Can you work these out from the model? Positions are in its coordinate system, mm. Face numbers are marked on the shaded views. A direction names the side the tool comes from. Coordinates: 2 decimals unless noted, no trailing zeros. Order: outer loops, then holes, each group sorted by start corner. A loop starts at its lowest first (then second) coordinate and runs counter-clockwise, first axis right, second up.
Autodesk Inventor part; units mm, degrees
ref_plane "Work Plane1" through (76.2, 0, 0) normal (1, 0, 0) x (0, 1, 0)
ref_plane "Work Plane4" through (63.5, 0, 0) normal (1, 0, 0) x (0, 1, 0)
ref_plane "XZ Plane" through (0, 0, 0) normal (0, 1, 0) x (-1, 0, 0)
sketch "Sketch1" plane through (0, 0, 0) normal (0, 0, 1) x (1, 0, 0)
  line L0 (107.721093, 0) -> (-76.2, 0)
  line L1 (-76.2, 0) -> (-76.2, -12.7)
  line L2 (-76.2, -12.7) -> (69.621093, -12.700026)
  line L3 (107.721093, -6.350016) -> (107.721093, 0)
  line L4 (107.721093, -6.350016) -> (69.621093, -12.700026)
  point P0 (0, 0)
  dimension "d19" = 183.92109
  dimension "d20" = 76.2
  dimension "d21" = 12.7
  dimension "d22" = 38.1
extrude "Extrusion2" add sketch "Sketch1" along normal blind 25.4
sketch "Sketch2" plane through (-76.2, 0, 0) normal (0, 1, 0) x (1, 0, 0)
  circle A0 centre (76.2, 0) radius 22.5
  dimension "d25" = 45
extrude "Extrusion3" cut sketch "Sketch2" against normal through all
mirror "Mirror1" about plane through (14.352169, -5.990033, 0) normal (0, 0, -1) of "Extrusion2", "Extrusion3"
sketch "Sketch4" plane through (-76.2, 0, 25.4) normal (0, 1, 0) x (1, 0, 0)
  circle A0 centre (38.1, 25.4) radius 3.81
  line L0 (-36.784219, 25.4) -> (220.705311, 25.4)
  point P0 (76.2, 25.4)
  dimension "d13" = 7.62
  dimension "d39" = 38.1
extrude "Extrusion5" add sketch "Sketch4" along normal blind 7.62
ref_plane "Work Plane1" through (76.2, 0, 0) normal (1, 0, 0) x (0, 1, 0)
sketch "Sketch10" plane through (69.621093, -12.700026, -25.4) normal (-0.0000002, -1, 0) x (1, -0.0000002, 0)
  line L0 (-69.621095, 36.62532) -> (38.099999, 36.62532)
  line L1 (-69.621095, 14.17468) -> (38.1, 14.17468)
  circle A0 centre (-69.621095, 25.4) radius 11.22532
  line L2 (-69.621095, 36.62532) -> (-69.621095, 14.17468) construction
  line L3 (38.099999, 0) -> (38.099999, 50.8) construction
  line L4 (38.099999, 36.62532) -> (38.1, 14.17468)
  point P0 (-69.621095, 25.4)
extrude "Extrusion11" cut sketch "Sketch10" against normal mid plane 15.24
ref_plane "Work Plane4" through (63.5, 0, 0) normal (1, 0, 0) x (0, 1, 0)
sketch "Sketch5" plane through (76.2, 0, 0) normal (1, 0, 0) x (0, 1, 0)
  line L0 (-1.5875, -10.237854) -> (9.525, -10.237854)
  line L1 (9.525, -10.237854) -> (9.525, 10.237854)
  line L2 (9.525, 10.237854) -> (-1.5875, 10.237854)
  line L3 (-1.5875, 10.237854) -> (-1.5875, -10.237854)
  line L4 (9.525, -7.62) -> (0, -7.62)
  line L5 (0, -7.62) -> (0, 7.62)
  line L6 (0, 7.62) -> (9.525, 7.62)
  line L7 (9.525, 7.62) -> (9.525, -7.62)
  line L8 (0, 25.4) -> (0, -25.4)
  line L9 (9.525, -7.62) -> (6.5, -7.62)
  line L10 (6.5, -7.62) -> (6.5, -4.62)
  line L11 (6.5, -4.62) -> (9.525, -4.62)
  line L12 (9.525, -4.62) -> (9.525, -7.62)
  line L13 (9.525, 7.62) -> (6.5, 7.62)
  line L14 (6.5, 7.62) -> (6.5, 4.62)
  line L15 (6.5, 4.62) -> (9.525, 4.62)
  line L16 (9.525, 4.62) -> (9.525, 7.62)
  point P0 (0, 0)
  point P1 (0, 0)
  point P2 (9.525, 0)
  dimension "d14" = 15.24
  dimension "d50" = 6.5
  dimension "d51" = 3
  dimension "d52" = 3
extrude "Extrusion6" add sketch "Sketch5" along normal blind 20 contours L3 L2 L8 L5 L0 | L8 L4 L1 L0 | L2 L1 L6 L8 | L4 L10 L11 L1 | L6 L1 L15 L14
fillet "Fillet1" radius 0.635 4 edges at (96.2, 9.525, 7.4289) (76.2, 9.525, 7.4289) (76.2, 9.525, -7.4289) (96.2, 9.525, -7.4289)
chamfer "Chamfer1" distance 12.7 angle 45 2 edges at (-76.2, -6.35, -25.4) (-76.2, -6.35, 25.4)
sketch "Sketch11" plane through (63.5, 0, 0) normal (1, 0, 0) x (0, 1, 0)
  line L0 (-5.080017, 11.22532) -> (-12.700026, 11.22532)
  ellipse E0 centre (-5.080014, 0) end of major axis (-5.080014, -22.5) minor radius 0.000004 (-5.080017, 11.22532) -> (-5.080017, -11.22532) ccw
  line L1 (-12.700026, -11.22532) -> (-5.080017, -11.22532)
  line L2 (-12.700026, 11.22532) -> (-6.350016, 11.22532)
  line L3 (-6.350016, 11.22532) -> (-5.080033, 11.22532)
  line L4 (-5.080033, 11.22532) -> (-5.080033, -11.22532)
  line L5 (-6.350016, -11.22532) -> (-12.700026, -11.22532)
  arc A0 (-12.700026, 11.22532) -> (-12.700026, -11.22532) centre (-10.847911, 0) ccw
  circle A1 centre (-15.875014, 0) radius 2.54
  ellipse E1 centre (-12.700014, 0) end of major axis (-12.700014, 22.5) minor radius 0.000004 (-12.700026, -11.22532) -> (-12.700026, 11.22532) ccw
  point P0 (0, 0)
  dimension "d48" = 3.175
  dimension "d49" = 5.08
extrude "Extrusion12" add sketch "Sketch11" along normal mid plane 12.7
sketch "Sketch12" plane through (107.721093, 0, 25.4) normal (0, 1, 0) x (1, 0, 0)
  line L0 (-171.221093, 50.8) -> (0, 50.8)
  line L1 (0, 0) -> (0, 50.8)
  line L2 (-171.221093, 0) -> (0, 0)
  line L3 (0, 25.4) -> (-107.721093, 25.4) construction
  ellipse E0 centre (-63.5, 25.4) end of major axis (0, 25.4) minor radius 25.4 (-63.5, 0) -> (-63.5, 50.8) ccw
extrude "Extrusion13" cut sketch "Sketch12" against normal through all
properties part number "Guide" material "UHMW, Black"
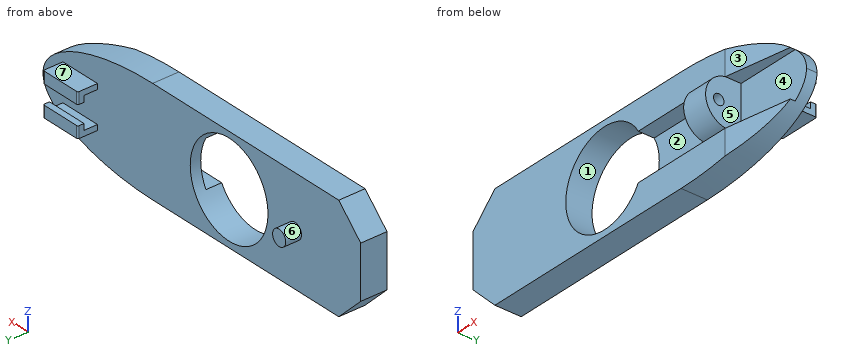
1. Imagine slicing it at B-B on x = 0. Please give me the cut outline in (y, z), then the cut area to 3 significant figures.
Completed:
outline: (-12.7, -25.4) - (0, -25.4) - (0, -22.5) - (-12.7, -22.5) - close; (-12.7, 22.5) - (0, 22.5) - (0, 25.4) - (-12.7, 25.4) - close
area: 73.7 mm2
2. I'm going to push flat-ended pins straight in: pin 1 (3 mm diameter, centred on y = -12, z = -20, fed in from -X); pin 2 (5 mm diameter, centred on y = -16, z = -4.5, fed in from +X); pin 3 (5 mm diameter, centred on x = 89, y = 3, fed in from -Z); pin 4 (4.5 mm diameter, centred on y = -15.88, z = 0, fed in from -X). Where does each tip first touch, or does it pass through?
Completed:
pin 1: stops at x = -70.4
pin 2: stops at x = 69.85
pin 3: stops at z = -10.24
pin 4: passes through
3. Imagine slicing it at A-A on y = 3. Please give me the cut outline in (x, z), then the cut area to 3 significant figures.
Completed:
outline: circle Ø7.62 at (-38.1, 0); (76.2, -10.24) - (96.2, -10.24) - (96.2, -7.62) - (76.2, -7.62) - close; (76.2, 7.62) - (96.2, 7.62) - (96.2, 10.24) - (76.2, 10.24) - close
area: 150 mm2
4. On a 3-axis mill with a long thin cutter (end or side, diameter ignored), from which of +Z, -Z, +X, -X, +Y, -Y can I reach the whole of each face in a straight line? I mean the marked faces 5, 6 and 7. Say none if no direction works.
Completed:
face 5: +X, -Y
face 6: +Y
face 7: +Z, +X, -X, +Y
5. Imagine slicing it at C-C on x = -38.1. Please give me the cut outline in (y, z), then the cut area to 3 significant figures.
Completed:
outline: (-12.7, -25.4) - (0, -25.4) - (0, -3.81) - (7.62, -3.81) - (7.62, 3.81) - (0, 3.81) - (0, 25.4) - (-12.7, 25.4) - close
area: 703 mm2
6. Thinking about a two-plate mould opening in X: for the marked faces 1, 2, 3 and 4, which applies, pulls with the +X half, pulls with the -X half, needs draft (parallel to the pull), parting line crosses it, or undercut?
Completed:
face 1: undercut
face 2: undercut
face 3: pulls with the +X half
face 4: needs draft
7. Please list where these lines run through material, in increasing order: probe 1 along X at (y, z) = (-5, 0); probe 2 along Z at (x, y) = (0, -8.5); probe 3 along X at (y, z) = (-5.5, 0).
Completed:
probe 1: x = -76.2 to -22.5, 22.5 to 107.72
probe 2: z = -25.4 to -22.5, 22.5 to 25.4
probe 3: x = -76.2 to -22.5, 57.15 to 69.85
